The listing builds one solid part. Answer for the finished solid, in the listing's coordinates (mm). A direction names the side the tool comes from. Give positions to 0.01 mm unless a question says otherwise; leave off trailing zeros. Loops run counter-clockwise (first coordinate to the right, second up) from the corner with the lowest first, then second, coordinate; pieces in that order, holes last.
Item 1: Section B-B, the plane x = 0 is taken. Give the vertices of the cut face in (y, z), and give its area (4 significant figures).
Item 2: A tool of negligible diameter and unlimited length cuts with its end or side. For faces 1 (the face through (0, 13.25, 3)), 2 (the face through (14, 0, 5)), from which of +Z, -Z, +X, -X, +Y, -Y can it reach the whole face along a straight path? Write none if from no direction.
Item 3: Section A-A, the plane y = 0 is taken. Give the vertices of the cut face in (x, z), and give its area (4 significant figures).
Item 4: Section D-D, the plane x = 6.5 is taken. Give the vertices of the cut face in (y, z).
Item 5: The mould has two halves that part along X. Classify faces 3 (the face through (12.25, 0, 3)), 4 (the face through (14, 0, 0)), 5 (the face through (-6.94, -31.24, 2.46)): pulls with the +X half, pulls with the -X half, needs draft (parallel to the pull), parting line crosses it, or undercut.
Item 6: Section C-C, the plane z = 3.9 is taken. Give the number of separate pieces and of enclosed holes in the cut face, and give its area (3 significant figures).
Item 7: Consider line 1 along X through (y, z) = (-19, 1.65); line 2 along X through (y, z) = (-13, 1.6); line 3 along X through (y, z) = (1, 2.6). Determine where each line is inside the solid, lowest interval first.
Item 8: Each of these flat-tipped pins is pushed along its axis until it touches: pin 1 Ø1.5 at (x, y) = (-28, 0) entering from -Z; pin 2 Ø1.5 at (x, z) = (-1, 3) entering from +Y; pin 3 Ø3 at (x, z) = (-19.5, 2) entering from +Y; pin 4 Ø1.5 at (y, z) = (-2.5, 3.5) entering from -X. Where does it stop, or does it pass through?
from build123d import *

# Parameters (mm, degrees)
CROQUIS1_R              = 32
SALIENTE_EXTRUIR1_DEPTH = 5
CROQUIS2_R              = 1.25
CORTAR_EXTRUIR1_DEPTH   = 46.530209751
CROQUIS3_W              = 24.5
CROQUIS3_H              = 26.5
CORTAR_EXTRUIR2_DEPTH   = 10


with BuildPart() as part:
    # Croquis1 → Saliente-Extruir1 (new body)
    with BuildSketch(Plane.XY):
        Circle(CROQUIS1_R)
    extrude(amount=SALIENTE_EXTRUIR1_DEPTH)

    # Croquis2 → Cortar-Extruir1 (cut, through all)
    with BuildSketch(Plane.XY.offset(5)):
        with Locations((0, 28)):
            Circle(CROQUIS2_R)
        with Locations((19.798989873, 19.798989873)):
            Circle(CROQUIS2_R)
        with Locations((28, 0)):
            Circle(CROQUIS2_R)
        with Locations((19.798989873, -19.798989873)):
            Circle(CROQUIS2_R)
        with Locations((0, -28)):
            Circle(CROQUIS2_R)
        with Locations((-19.798989873, -19.798989873)):
            Circle(CROQUIS2_R)
        with Locations((-28, 0)):
            Circle(CROQUIS2_R)
        with Locations((-19.798989873, 19.798989873)):
            Circle(CROQUIS2_R)
    extrude(amount=-CORTAR_EXTRUIR1_DEPTH, mode=Mode.SUBTRACT)

    # Croquis3 → Cortar-Extruir2 (cut)
    with BuildSketch(Plane.XY.offset(5)):
        Rectangle(CROQUIS3_W, CROQUIS3_H)
    extrude(amount=-CORTAR_EXTRUIR2_DEPTH, mode=Mode.SUBTRACT)


solid = part.part
Worked answers:
1. outline: (-32, 0) - (-29.25, 0) - (-29.25, 5) - (-32, 5) - close; (-26.75, 0) - (-13.25, 0) - (-13.25, 5) - (-26.75, 5) - close; (13.25, 0) - (26.75, 0) - (26.75, 5) - (13.25, 5) - close; (29.25, 0) - (32, 0) - (32, 5) - (29.25, 5) - close
1. area: 162.5 mm2
2. face 1: +Z, -Z
2. face 2: +Z, +X, -X, +Y, -Y
3. outline: (-32, 0) - (-29.25, 0) - (-29.25, 5) - (-32, 5) - close; (-26.75, 0) - (-12.25, 0) - (-12.25, 5) - (-26.75, 5) - close; (12.25, 0) - (26.75, 0) - (26.75, 5) - (12.25, 5) - close; (29.25, 0) - (32, 0) - (32, 5) - (29.25, 5) - close
3. area: 172.5 mm2
4. outline: (-31.33, 0) - (-13.25, 0) - (-13.25, 5) - (-31.33, 5) - close; (13.25, 0) - (31.33, 0) - (31.33, 5) - (13.25, 5) - close
5. face 3: undercut
5. face 4: needs draft
5. face 5: parting line crosses it
6. separate pieces: 1
6. enclosed holes: 9
6. area: 2,530 mm2
7. line 1: x = -25.75 to -20.76, -18.84 to 18.84, 20.76 to 25.75
7. line 2: x = -29.24 to -12.25, 12.25 to 29.24
7. line 3: x = -31.98 to -28.75, -27.25 to -12.25, 12.25 to 27.25, 28.75 to 31.98
8. pin 1: passes through
8. pin 2: stops at y = 32
8. pin 3: stops at y = 26.46
8. pin 4: stops at x = -31.95
